Here's how the part is built. I have some questions about the finished solid (model axes, mm). Face numbers are marked on the shaded views. A direction names the side the tool comes from. Give positions to 0.01 mm unless a question says otherwise; leave off trailing zeros. Loops run counter-clockwise (first coordinate to the right, second up) from the corner with the lowest first, then second, coordinate; pieces in that order, holes last. Notation, with made-up numbers: M 81.5,-25 L 112.5,-25 A14 ccw 112.5,-18 Z; hole C 44,82 d7. An arc over 180 degrees is marked long. Write item = value, one per line. Start each with the question number.
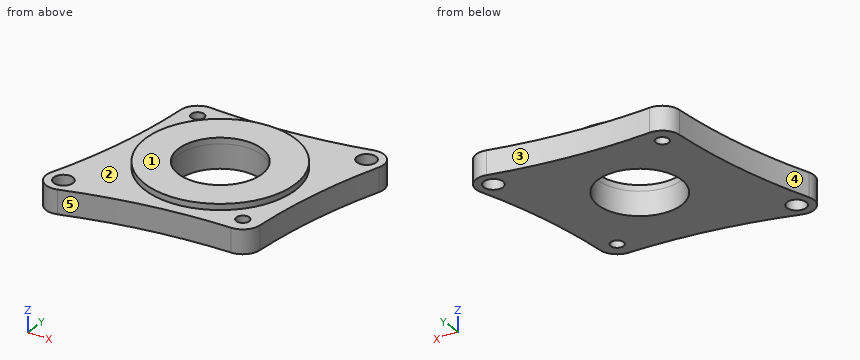
```python
from build123d import *
from build123d.topology import SkipClean

# Parameters (mm, degrees)
BOSS_EXTRUDE1_DEPTH          = 6.35
F_7_8_0_875_DIAMETER_HOLE1_D = 22.225
F_10_CLEARANCE_HOLE1_D       = 5.1054
F_8_32_TAPPED_HOLE1_D        = 3.4544
SKETCH33_R                   = 19.939
SKETCH33_R_2                 = 11.1125
BOSS_EXTRUDE3_DEPTH          = 1.5875


with BuildPart() as part:
    # Sketch1 → Boss-Extrude1 (new body)
    with BuildSketch(Plane.XY):
        with BuildLine():
            ThreePointArc((29.724646249, 19.656342437), (28.792029634, 24.206107761), (24.36391271, 25.606792867))
            ThreePointArc((24.36391271, 25.606792867), (3.704744399, 22.428476482), (-17.196740725, 22.25283495))
            ThreePointArc((-17.196740725, 22.25283495), (-20.654876788, 21.06765451), (-22.254232731, 17.780494905))
            ThreePointArc((-22.254232731, 17.780494905), (-24.94278341, -2.733369886), (-30.522874393, -22.655958523))
            ThreePointArc((-30.522874393, -22.655958523), (-29.526294957, -27.367332021), (-24.868197962, -28.588947016))
            ThreePointArc((-24.868197962, -28.588947016), (-3.918964321, -23.852830981), (17.5, -22.2625))
            ThreePointArc((17.5, -22.2625), (20.756780188, -20.974879718), (22.252512093, -17.808277557))
            ThreePointArc((22.252512093, -17.808277557), (24.749635252, 1.17113371), (29.724646249, 19.656342437))
        make_face()
    extrude(amount=BOSS_EXTRUDE1_DEPTH)

    # 7/8 (0.875) Diameter Hole1 (through all)
    with Locations(Plane.XY.offset(6.35)):
        with Locations((0, 0)):
            Hole(F_7_8_0_875_DIAMETER_HOLE1_D / 2)

    # #10 Clearance Hole1 (through all)
    with Locations(Plane.XY.offset(6.35)):
        with Locations((25.385765971, 21.137420428), (-26.207516439, -24.204234926)):
            Hole(F_10_CLEARANCE_HOLE1_D / 2)

    # #8-32 Tapped Hole1 (through all)
    with Locations(Plane.XY.offset(6.35)):
        with Locations((17.5, -17.5), (-17.5, 17.5)):
            Hole(F_8_32_TAPPED_HOLE1_D / 2)

    # Sketch33 → Boss-Extrude3 (add)
    with SkipClean():  # the faces are left unmerged after this step: merging them gives an invalid solid
        with BuildSketch(Plane.XY.offset(6.35)):
            Circle(SKETCH33_R)
            Circle(SKETCH33_R_2, mode=Mode.SUBTRACT)
        extrude(amount=BOSS_EXTRUDE3_DEPTH)
    add(part.part.scale(1), mode=Mode.REPLACE)  # the faces are merged on a copy


solid = part.part
```
Q1. On a 3-axis mill with a long thin cutter (end or side, diameter ignored), from which of +Z, -Z, +X, -X, +Y, -Y can I reach the whole of each face in a straight line? I mean the marked faces 1 and 2. Say none if no direction works.
Q2. Will these pins go through, and if not, where does the flat tip stop? pin 1 (6 mm diameter, centred on x = -7, y = -17.5, fed in from -Z); pin 2 (4 mm diameter, centred on x = 2.5, z = 5, fed in from +Y); pin 3 (1 mm diameter, centred on x = 20.5, z = 1.5, fed in from -Y); pin 4 (1 mm diameter, centred on x = -16.5, z = 1, fed in from +Y).
Q3. If we section it at D-D, the plane y = 14: List the corners of the cut face in (x, z) for me, then the cut area to 3 significant figures.
Q4. We'd pull the mould along X, two halves only. Please class the marked faces 3, 4 and 5: pulls with the +X half, pulls with the -X half, needs draft (parallel to the pull), parting line crosses it, or undercut.
Q5. If we section it at B-B, the plane y = 0: List the corners of the cut face in (x, z) for me.
Q6. If we section it at A-A, the plane x = 8.5: List the corners of the cut face in (y, z) for me.
Q7. If we section it at C-C, the plane z = 3.75: List the corners of the cut face in (x, y) for me (1 decimal).
Q8. If I drill on line 1 along Y through (x, z) = (0, 6.9); line 2 along Z through (x, y) = (21.5, -6); line 3 along X through (y, z) = (0, 2.5), over which ranges is the centre line in solid material (lowest first)?
Resolved:
q1.face_1 = +Z, +X, -X, +Y, -Y
q1.face_2 = +Z
q2.pin_1 = 0
q2.pin_2 = 22.49
q2.pin_3 = -21.55
q2.pin_4 = 22.24
q3.outline = M -22.53,0 L 27.92,0 L 27.92,6.35 L 14.2,6.35 L 14.2,7.94 L -14.2,7.94 L -14.2,6.35 L -22.53,6.35 Z
q3.area = 365 mm²
q4.face_3 = undercut
q4.face_4 = pulls with the -X half
q4.face_5 = pulls with the +X half
q5.outline = M -24.41,0 L -11.11,0 L -11.11,7.94 L -19.94,7.94 L -19.94,6.35 L -24.41,6.35 Z; M 11.11,0 L 24.52,0 L 24.52,6.35 L 19.94,6.35 L 19.94,7.94 L 11.11,7.94 Z
q6.outline = M -22.54,0 L -7.16,0 L -7.16,7.94 L -18.04,7.94 L -18.04,6.35 L -22.54,6.35 Z; M 7.16,0 L 22.9,0 L 22.9,6.35 L 18.04,6.35 L 18.04,7.94 L 7.16,7.94 Z
q7.outline = M -30.5,-22.7 A4.6 ccw -24.9,-28.6 A145 cw 17.5,-22.3 A4.8 ccw 22.3,-17.8 A145 cw 29.7,19.7 A4.6 ccw 24.4,25.6 A145 cw -17.2,22.3 A4.8 ccw -22.3,17.8 A145 cw Z; hole C -26.2,-24.2 d5.1; hole C -17.5,17.5 d3.5; hole C 0,0 d22.2; hole C 17.5,-17.5 d3.5; hole C 25.4,21.1 d5.1
q8.line_1 = -19.94 to -11.11, 11.11 to 19.94
q8.line_2 = 0 to 6.35
q8.line_3 = -24.41 to -11.11, 11.11 to 24.52
